Check sheet for the modelled part. Datum: model origin and axes. Units: mm. A direction names the side the tool comes from. Round coordinates to 2 decimals unless told otherwise and drop trailing zeros. Write each loop counter-clockwise with the first axis right and the second up, starting at its lowest first coordinate (ties: lowest second). Pieces come first, ordered by that corner, then holes. Notation, with made-up numbers: (-32.5, 25.25) -> (-15.5, 25.25) arc R36 ccw to (-15.5, 63.25) -> close; hole circle Ø6 at (86, 85). An arc over 180 degrees is marked (long way). One line per item, written item: value. Start each with the question number.
```python
from build123d import *

# Parameters (mm, degrees)
SKETCH1_W                      = 4.572
SKETCH1_H                      = 28.575
SKETCH2_R                      = 14.2875
BOSS_EXTRUDE1_DEPTH            = 0.889
SKETCH3_R                      = 12.9794
BOSS_EXTRUDE2_DEPTH            = 0.8128
BOSS_EXTRUDE2_TAPER            = 45
SKETCH4_R                      = 12.1666
BOSS_EXTRUDE3_DEPTH            = 18.2372
SKETCH5_R                      = 14.2875
BOSS_EXTRUDE4_DEPTH            = 0.889
CUT_EXTRUDE1_DEPTH             = 26.4
F_6_0_204_DIAMETER_HOLE1_D     = 5.1816
F_6_0_204_DIAMETER_HOLE1_DEPTH = 24.511
CHAMFER1_SIZE                  = 0.254


with BuildPart() as part:
    # Sketch1 → Revolve1 (revolve)
    with BuildSketch(Plane(origin=(0, 0, 0), x_dir=(-1, 0, 0), z_dir=(0, 0, -1))):
        with Locations((16.210066246, 14.2875)):
            Rectangle(SKETCH1_W, SKETCH1_H)
    revolve(axis=Axis((-13.924066246, 0, 0), (-1, 0, 0)))

    # Sketch2 → Boss-Extrude1 (add)
    with BuildSketch(Plane(origin=(-13.924066246, 0, 0), x_dir=(0, 0, -1), z_dir=(1, 0, 0))):
        Circle(SKETCH2_R)
    extrude(amount=BOSS_EXTRUDE1_DEPTH)

    # Sketch3 → Boss-Extrude2 (add)
    with BuildSketch(Plane(origin=(-13.035066246, 0, 0), x_dir=(0, 0, -1), z_dir=(1, 0, 0))):
        Circle(SKETCH3_R)
    extrude(amount=BOSS_EXTRUDE2_DEPTH, taper=BOSS_EXTRUDE2_TAPER)

    # Sketch4 → Boss-Extrude3 (add)
    with BuildSketch(Plane(origin=(-12.222266246, 0, 0), x_dir=(0, 0, -1), z_dir=(1, 0, 0))):
        Circle(SKETCH4_R)
    extrude(amount=BOSS_EXTRUDE3_DEPTH)

    # Sketch5 → Boss-Extrude4 (add)
    with BuildSketch(Plane.ZY.offset(18.496066246)):
        Circle(SKETCH5_R)
    extrude(amount=BOSS_EXTRUDE4_DEPTH)

    # Sketch6 → Cut-Extrude1 (cut, through all)
    with BuildSketch(Plane.ZY.offset(19.385066246)):
        Polygon((0, 7.361657812), (-6.3754, 3.680818906), (-6.3754, -3.680858906), (0, -7.361697812), (6.3754, -3.680858906), (6.3754, 3.680818906), align=None)
    extrude(amount=-CUT_EXTRUDE1_DEPTH, mode=Mode.SUBTRACT)

    # #6 (0.204) Diameter Hole1
    with Locations(Plane.ZY.offset(18.496066246)):
        with Locations((11.90625, 20.622229928), (-23.8125, 0), (11.90625, -20.622229928), (-11.90625, -20.622229928), (-11.90625, 20.622229928), (23.8125, 0)):
            Hole(F_6_0_204_DIAMETER_HOLE1_D / 2, depth=F_6_0_204_DIAMETER_HOLE1_DEPTH)

    # Chamfer1
    chamfer1_edges = [part.edges().sort_by_distance(p)[0] for p in [
        (6.014933754, 0, 12.1666),
        (-19.385066246, 0, -14.2875),
        (-18.496066246, -28.575, 0),
        (-13.924066246, -28.575, 0),
        (-13.035066246, 0, 14.2875),
    ]]
    chamfer(chamfer1_edges, length=CHAMFER1_SIZE)


solid = part.part
```
1. Access from +Z, -Z, +X, -X, +Y, -Y to the whole of each face (thin tool, end or side, straight path). Record for faces 4 (the face through (-13.924, 13, -7)), 5 (the face through (6.015, -5, -5)), 6 (the face through (-6.86, 5.55, -3.14)), 7 (the face through (-18.809, 0.628, -14.274)).
2. Material ranges on probe 1 along X at (y, z) = (14.5, -13); probe 2 along Z at (x, y) = (4.5, -2.5); probe 3 along Y at (x, z) = (-17.5, 0) (3 decimals), recorded low to high.
3. Cross-section at B-B (y = 0). Give the number of separate pieces and of enclosed holes in the cut face, plus the area to 3 significant figures.
4. Release check for a two-part mould opening along Y. For faces 1 (the face through (-19.385, -6, 3)), 2 (the face through (-6.863, 5.495, 3.232)), 3 (the face through (-16.239, -28.547, -1.256)) record: +Y half, -Y half, draft (parallel to the pull), parting line (faces both ways), or undercut.
5. Cross-section at A-A (x = -10.75). Record the cut outline in (y, z).
6. Depth check by flat-ended pin: pin 1 Ø1.5 at (x, y) = (-10.5, 2) entering from +Z; pin 2 Ø6.5 at (y, z) = (20.62, 11.91) entering from +X; pin 3 Ø1 at (x, z) = (-1, 10) entering from +Y. Enter the tip coordinate at first touch or a pass-through.
Working result:
1. face 4: +X
1. face 5: +Z, -Z, +X, +Y, -Y
1. face 6: +X, -X
1. face 7: -X
2. probe 1: x = -18.5 to -13.92
2. probe 2: z = -11.91 to -6.38, 6.38 to 11.91
2. probe 3: y = -28.575 to -7.362, 7.362 to 28.575
3. separate pieces: 4
3. enclosed holes: 0
3. area: 405 mm^2
4. face 1: draft
4. face 2: undercut
4. face 3: parting line
5. outline: circle Ø24.33 at (0, 0); hole (-7.36, 0) -> (-3.68, -6.38) -> (3.68, -6.38) -> (7.36, 0) -> (3.68, 6.38) -> (-3.68, 6.38) -> close
6. pin 1: stops at z = 12.1
6. pin 2: stops at x = -13.92
6. pin 3: stops at y = 7.6
